Check sheet for the modelled part. Datum: model origin and axes. Units: mm. A direction names the side the tool comes from. Give positions to 0.01 mm unless a question says otherwise; leave off trailing zeros. Loops run counter-clockwise (first coordinate to the right, second up) from the corner with the lowest first, then second, coordinate; pieces in that order, holes last.
```python
from build123d import *

# Parameters (mm, degrees)
SKETCH2_R               = 1.8
CUT_EXTRUDE1_DEPTH      = 10
SKETCH3_W               = 5.6
SKETCH3_H               = 10.691433847
CUT_EXTRUDE2_DEPTH      = 2.4
BOSS_EXTRUDE1_DEPTH     = 2.5
SKETCH5_R               = 1.8
CUT_EXTRUDE3_DEPTH      = 92.554113097
SKETCH6_W               = 5.6
SKETCH6_H               = 10.168713577
SKETCH6_W_2             = 10.168713577
SKETCH6_H_2             = 5.6
CUT_EXTRUDE4_DEPTH      = 2.4
CUT_EXTRUDE5_DEPTH      = 95.516678422
CUT_EXTRUDE5_DEPTH_BACK = 95.516678422
SKETCH7_W               = 158.937204397
SKETCH7_H               = 29.823360181
SKETCH8_R               = 53.05
CUT_EXTRUDE6_DEPTH      = 3.1
CHAMFER1_SIZE           = 1
CHAMFER3_SIZE           = 0.5
CHAMFER4_SIZE           = 0.5
CHAMFER5_SIZE           = 1


with BuildPart() as part:
    # Sketch1 → Revolve1 (revolve)
    with BuildSketch(Plane(origin=(0, 0, 0), x_dir=(1, 0, 0), z_dir=(0, 1, 0))):
        Polygon((43.05, 0), (43.05, 5.5), (40.025, 5.5), (40.025, 8.05), (33.75, 8.05), (33.75, 11.55), (47.85, 11.55), (47.85, 26.55), (33.75, 26.55), (33.75, 31.55), (46.9, 31.55), (46.9, 29.55), (50.35, 29.55), (50.35, 24.55), (53.5, 24.55), (53.5, 31.55), (55, 31.55), (55, 20.475), (63, 20.475), (63, 10.475), (55, 10.475), (55, 0), align=None)
    revolve(axis=Axis((0, 0, 39.851832449), (0, 0, -1)))

    # Sketch2 → Cut-Extrude1 (cut)
    with BuildSketch(Plane.XY):
        with Locations((0, 50)):
            Circle(SKETCH2_R)
        with Locations((43.301270189, 25)):
            Circle(SKETCH2_R)
        with Locations((43.301270189, -25)):
            Circle(SKETCH2_R)
        with Locations((0, -50)):
            Circle(SKETCH2_R)
        with Locations((-43.301270189, -25)):
            Circle(SKETCH2_R)
        with Locations((-43.301270189, 25)):
            Circle(SKETCH2_R)
    extrude(amount=-CUT_EXTRUDE1_DEPTH, mode=Mode.SUBTRACT)

    # Sketch3 → Cut-Extrude2 (cut)
    with BuildSketch(Plane.XY.offset(-5)):
        with Locations((0, 52.545716924)):
            Rectangle(SKETCH3_W, SKETCH3_H)
        Polygon((51.535452373, 26.520845793), (48.735452373, 31.370588054), (39.476399059, 26.024871131), (42.276399059, 21.175128869), align=None)
        Polygon((48.735452373, -31.370588054), (51.535452373, -26.520845793), (42.276399059, -21.175128869), (39.476399059, -26.024871131), align=None)
        with Locations((0, -52.545716924)):
            Rectangle(SKETCH3_W, SKETCH3_H)
        Polygon((-51.535452373, -26.520845793), (-48.735452373, -31.370588054), (-39.476399059, -26.024871131), (-42.276399059, -21.175128869), align=None)
        Polygon((-48.735452373, 31.370588054), (-51.535452373, 26.520845793), (-42.276399059, 21.175128869), (-39.476399059, 26.024871131), align=None)
    extrude(amount=-CUT_EXTRUDE2_DEPTH, mode=Mode.SUBTRACT)

    # Sketch4 → Boss-Extrude1 (add)
    with BuildSketch(Plane.XY.offset(-5.5)):
        with BuildLine():
            Line((-2.45, 42.980228012), (-2.45, 39.949945244))
            ThreePointArc((-2.45, 39.949945244), (0, 40.025), (2.45, 39.949945244))
            Line((2.45, 39.949945244), (2.45, 42.980228012))
            ThreePointArc((2.45, 42.980228012), (0, 43.05), (-2.45, 42.980228012))
        make_face()
    extrude(amount=BOSS_EXTRUDE1_DEPTH)

    # Sketch5 → Cut-Extrude3 (cut, through all)
    with BuildSketch(Plane.XY.offset(-10.475)):
        with Locations((0, 59)):
            Circle(SKETCH5_R)
        with Locations((59, 0)):
            Circle(SKETCH5_R)
        with Locations((0, -59)):
            Circle(SKETCH5_R)
        with Locations((-59, 0)):
            Circle(SKETCH5_R)
    extrude(amount=-CUT_EXTRUDE3_DEPTH, mode=Mode.SUBTRACT)

    # Sketch6 → Cut-Extrude4 (cut)
    with BuildSketch(Plane.XY.offset(-16.775)):
        with Locations((0, 61.284356789)):
            Rectangle(SKETCH6_W, SKETCH6_H)
        with Locations((61.284356789, 0)):
            Rectangle(SKETCH6_W_2, SKETCH6_H_2)
        with Locations((0, -61.284356789)):
            Rectangle(SKETCH6_W, SKETCH6_H)
        with Locations((-61.284356789, 0)):
            Rectangle(SKETCH6_W_2, SKETCH6_H_2)
    extrude(amount=-CUT_EXTRUDE4_DEPTH, mode=Mode.SUBTRACT)

    # Sketch7 → Cut-Extrude5 (cut, two sides: drawn at the far end of the back side and taken through both)
    with BuildSketch(Plane(origin=(0, 0, 0), x_dir=(1, 0, 0), z_dir=(0, 1, 0)).offset(-CUT_EXTRUDE5_DEPTH_BACK)):
        with Locations((-3.919975894, 0.56331991)):
            Rectangle(SKETCH7_W, SKETCH7_H)
    extrude(amount=CUT_EXTRUDE5_DEPTH + CUT_EXTRUDE5_DEPTH_BACK, mode=Mode.SUBTRACT)

    # Sketch8 → Cut-Extrude6 (cut)
    with BuildSketch(Plane.XY.offset(-15.475)):
        Circle(SKETCH8_R)
    extrude(amount=-CUT_EXTRUDE6_DEPTH, mode=Mode.SUBTRACT)

    # Chamfer1
    chamfer1_edges = [part.edges().sort_by_distance(p)[0] for p in [
        (-55, 0, -20.475),
    ]]
    chamfer(chamfer1_edges, length=CHAMFER1_SIZE)

    # Chamfer3
    chamfer3_edges = [part.edges().sort_by_distance(p)[0] for p in [
        (-50.35, 0, -29.55),
    ]]
    chamfer(chamfer3_edges, length=CHAMFER3_SIZE)

    # Chamfer4
    chamfer4_edges = [part.edges().sort_by_distance(p)[0] for p in [
        (-53.5, 0, -31.55),
    ]]
    chamfer(chamfer4_edges, length=CHAMFER4_SIZE)

    # Chamfer5
    chamfer5_edges = [part.edges().sort_by_distance(p)[0] for p in [
        (-47.85, 0, -18.575),
    ]]
    chamfer(chamfer5_edges, length=CHAMFER5_SIZE)


solid = part.part
```
(1) Gauge pin test, flat ends, axial feed: pin 1 Ø1.9 at (x, z) = (58.5, -18) entering from +Y; pin 2 Ø1.5 at (y, z) = (-26.5, -25.5) entering from +X; pin 3 Ø6 at (y, z) = (17, -21) entering from +X. Record the tip position at first contact, or that the pin passes through.
(2) Release check for a two-part mould opening along Z. For faces 1 (the face through (-11.5, -51.79, -17)), 2 (the face through (-61, 0, -16.775)), 3 (the face through (14, -52, -15.475)) record: pulls with the +Z half, pulls with the -Z half, needs draft (parallel to the pull), parting line crosses it, or undercut.
(3) Section check A-A on x = 59. Record the boundary of the cut face in (y, z) (3 decimals), plus the area to 3 significant figures.
(4) Section check C-C on y = 0. Give the number of separate pieces and of enclosed holes in the cut face, plus the area to 3 significant figures.
(5) Access from +Z, -Z, +X, -X, +Y, -Y to the whole of each face (thin tool, end or side, straight path). Record for faces 4 (the face through (-33, 10, -26.55)), 5 (the face through (0, 61, -16.775)), 6 (the face through (61, 0, -19.175)), 7 (the face through (0, -61, -16.775)), 8 (the face through (24, -52, -20.475)).
(6) Material ranges on line 1 (Y direction, x = 0, z = -15.7); line 2 (X direction, y = 0, z = -27.7); line 3 (Y direction, x = 0, z = -20.2), recorded low to high.
Computed values:
1. pin 1: stops at y = 25.63
1. pin 2: stops at x = 48.6
1. pin 3: stops at x = 61.41
2. face 1: needs draft
2. face 2: undercut
2. face 3: pulls with the +Z half
3. outline: (-22.091, -20.475) - (-1.8, -20.475) - (-1.8, -19.175) - (-2.8, -19.175) - (-2.8, -16.775) - (-1.8, -16.775) - (-1.8, -15.475) - (-22.091, -15.475) - close; (1.8, -20.475) - (22.091, -20.475) - (22.091, -15.475) - (1.8, -15.475) - (1.8, -16.775) - (2.8, -16.775) - (2.8, -19.175) - (1.8, -19.175) - close
3. area: 198 mm2
4. separate pieces: 6
4. enclosed holes: 0
4. area: 309 mm2
5. face 4: +Z
5. face 5: +Y
5. face 6: +X
5. face 7: -Y
5. face 8: -Z
6. line 1: y = -63 to -60.8, -57.2 to -53.05, 53.05 to 57.2, 60.8 to 63
6. line 2: x = -55 to -53.5, -50.35 to -33.75, 33.75 to 50.35, 53.5 to 55
6. line 3: y = -63 to -60.8, -57.2 to -47.85, 47.85 to 57.2, 60.8 to 63
